```python
from build123d import *

# Parameters (mm, degrees)
SKETCH2_R           = 9.525
BOSS_EXTRUDE2_DEPTH = 4.7625
SKETCH5_R           = 3.175
BOSS_EXTRUDE3_DEPTH = 9.525
SKETCH6_R           = 3.175
CUT_EXTRUDE3_DEPTH  = 10.525


with BuildPart() as part:
    # Sketch2 → Boss-Extrude2 (new body, symmetric)
    with BuildSketch(Plane.XY):
        Circle(SKETCH2_R)
    extrude(amount=BOSS_EXTRUDE2_DEPTH, both=True)

    # Sketch5 → Boss-Extrude3 (add, symmetric)
    with BuildSketch(Plane.XY):
        Circle(SKETCH5_R)
    extrude(amount=BOSS_EXTRUDE3_DEPTH, both=True)

    # Sketch6 → Cut-Extrude3 (cut, through all)
    with BuildSketch(Plane(origin=(0, 0, 0), x_dir=(0, 0, -1), z_dir=(1, 0, 0))):
        Circle(SKETCH6_R)
    extrude(amount=-CUT_EXTRUDE3_DEPTH, mode=Mode.SUBTRACT)


solid = part.part
```
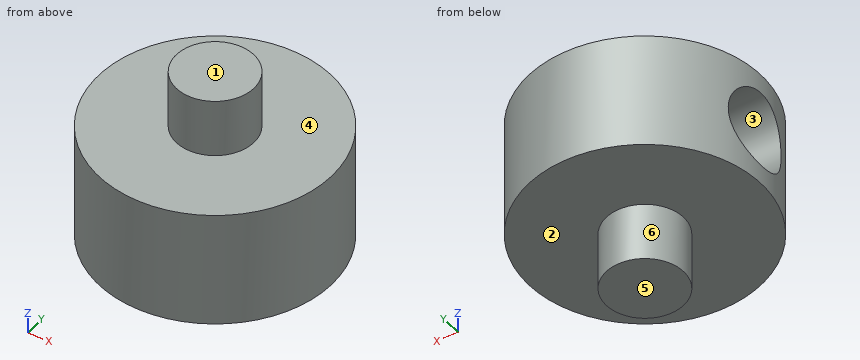
Geometry check sheet. Reference: the model listing, model coordinates, mm. Face numbers are marked on the shaded views. A direction names the side the tool comes from. Coordinates: 2 decimals unless noted, no trailing zeros. Write each loop counter-clockwise with the first axis right and the second up, starting at its lowest first coordinate (ties: lowest second). Pieces come first, ordered by that corner, then holes. Notation, with made-up numbers: M 9,-6.75 L 48,-6.75 A22 cw 48,20.25 Z; hole C 55,75 d9. An arc over 180 degrees is marked long. One line per item, written item: value. Start each with the question number.
(1) Tool access check on the marked faces 4, 5 and 6. Record the directions out of +Z, -Z, +X, -X, +Y, -Y that give a thin tool (end or side, any length) a straight path to the whole face; none if there is none.
(2) Scan lines: line 1 along Z through (x, y) = (-2.75, 7.25); line 2 along Z through (x, y) = (-2, 0) (3 decimals); line 3 along Y through (x, z) = (-2.5, 0) (3 decimals). Record each from-to range of solid material in increasing order. Write a range as [from, to].
(3) Release check for a two-part mould opening along Z. For the marked faces 1, 2 and 3 record: released by +Z, released by -Z, zero draft, split by the parting line, or undercut.
(4) Sectioned sample at A-A, the plane y = 0. Enter the section's corners in (x, z) (1 decimal), and give its area (3 significant figures).
(5) Sectioned sample at C-C, the plane z = 7.5. Enter the section's corners in (x, y) (3 decimals), and give its area (3 significant figures).
(6) Depth check by flat-ended pin: pin 1 (6 mm diameter, centred on x = -2, z = 1, fed in from -Y) (3 decimals); pin 2 (2 mm diameter, centred on x = -3, z = 4, fed in from +Y); pin 3 (1.5 mm diameter, centred on x = 1.5, y = -6.5, fed in from +Z); pin 4 (1.9 mm diameter, centred on y = -1, z = 1.5, fed in from -X). Enter the tip coordinate at first touch or a pass-through.
Filled sheet:
1. face 4: +Z
1. face 5: -Z, +X, -X, +Y, -Y
1. face 6: -Z
2. line 1: [-4.76, 4.76]
2. line 2: [-9.525, -3.175], [3.175, 9.525]
2. line 3: [-9.191, -3.175], [3.175, 9.191]
3. face 1: released by +Z
3. face 2: released by -Z
3. face 3: undercut
4. outline: M -9.5,-4.8 L -3.2,-4.8 L -3.2,-9.5 L 3.2,-9.5 L 3.2,-4.8 L 9.5,-4.8 L 9.5,4.8 L 3.2,4.8 L 3.2,9.5 L -3.2,9.5 L -3.2,4.8 L -9.5,4.8 L -9.5,3.2 L 0,3.2 L 0,-3.2 L -9.5,-3.2 Z
4. area: 181 mm²
5. outline: C 0,0 d6.35
5. area: 31.7 mm²
6. pin 1: y = -9.525
6. pin 2: y = 9.31
6. pin 3: z = 4.76
6. pin 4: x = 0
